Can you work these out from the model? Positions are in its coordinate system, mm. A direction names the side the tool comes from. Coordinates: 2 decimals unless noted, no trailing zeros. Order: outer loops, then holes, each group sorted by start corner. A loop starts at its lowest first (then second) coordinate and runs counter-clockwise, first axis right, second up. Notation, with made-up numbers: (0.25, 34) -> (8.25, 34) arc R12 cw to (8.25, 43) -> close; hole circle Ø4 at (50, 64.25). An arc over 180 degrees is marked (long way). Answer as CSV lines item,"result".
from build123d import *

# Parameters (mm, degrees)
F2_W     = 100
F2_H     = 100
F2_R     = 41
F2_R_2   = 26
F3_DEPTH = 20


with BuildPart() as f1:
    # F0 (on Front) → F1 (revolve)
    with BuildSketch(Plane.XZ):
        with BuildLine():
            Line((41, -5), (41, 0))
            Line((41, 0), (26, 0))
            ThreePointArc((26, 0), (22.464466, -1.464466), (21, -5))
            Line((21, -5), (21, -50))
            Line((21, -50), (26, -50))
            Line((26, -50), (26, -10))
            ThreePointArc((26, -10), (27.464466, -6.464466), (31, -5))
            Line((31, -5), (41, -5))
        make_face()
    revolve(axis=Axis((0, 0, -25.033533), (0, 0, -1)))

    # F2 (on face) → F3 (join)
    with BuildSketch(Plane.XY):
        Rectangle(F2_W, F2_H)
        Circle(F2_R, mode=Mode.SUBTRACT)
        Circle(F2_R)
        Circle(F2_R_2, mode=Mode.SUBTRACT)
    extrude(amount=-F3_DEPTH)


solid = f1.part
Q1. Which directions (+Z, -Z, +X, -X, +Y, -Y) give clear straight access to the entire face, cutting with the end or side of a thin tool? Please do faces 1 (the flat face through (-23, 23, -20)), 2 (the flat face through (-1.8, -21.3, -50)).
Solution:
face 1,"-Z"
face 2,"-Z, +X, -X, +Y, -Y"
Q2. If I drill on line 1 (Y direction, x = 0, z = -25); line 2 (Z direction, x = -45, y = 14), over which ranges is the centre line in solid material (lowest first)?
Solution:
line 1,"-26 to -21, 21 to 26"
line 2,"-20 to 0"
Q3. For P1, Ø25, axis at x = 0, y = 0, coming from the -Z side; P2, Ø4, axis at x = -17.5, z = -23, coming from the -Y side; P3, Ø12, axis at x = -10, z = -34, coming from the -Y side; P4, Ø4, axis at x = 30, y = 39, coming from the -Z side, each with a flat end and sliding along its axis, tell me the tip position at first contact or that it passes through.
Solution:
P1,"through"
P2,"y = -20.87"
P3,"y = -25.69"
P4,"z = -20"
Q4. Imagine slicing it at D-D (x = 42). List the corners of the cut face in (y, z) for me, and give its area (3 significant figures).
Solution:
outline,"(-50, -20) -> (50, -20) -> (50, 0) -> (-50, 0) -> close"
area,"2,000 mm2"
Q5. Imagine slicing it at A-A (x = 0). List the corners of the cut face in (y, z) for me, and give its area (3 significant figures).
Solution:
outline,"(-50, -20) -> (-26, -20) -> (-26, -50) -> (-21, -50) -> (-21, -5) arc R5 ccw to (-26, 0) -> (-50, 0) -> close; (21, -50) -> (26, -50) -> (26, -20) -> (50, -20) -> (50, 0) -> (26, 0) arc R5 ccw to (21, -5) -> close"
area,"1,450 mm2"
Q6. We'd pull the mould along Y, two halves only. Please class faces 3 (the flat face through (-23, 23, 0)), 4 (the cylindrical face through (20.03, -6.31, -27.82)), 5 (the cylindrical face through (-20.633, 15.821, -34.79)): pulls with the +Y half, pulls with the -Y half, needs draft (parallel to the pull), parting line crosses it, or undercut.
Solution:
face 3,"needs draft"
face 4,"undercut"
face 5,"parting line crosses it"
Q7. Imagine slicing it at C-C (z = -32). List the corners of the cut face in (x, y) for me, and give its area (3 significant figures).
Solution:
outline,"circle Ø52 at (0, 0); hole circle Ø42 at (0, 0)"
area,"738 mm2"
